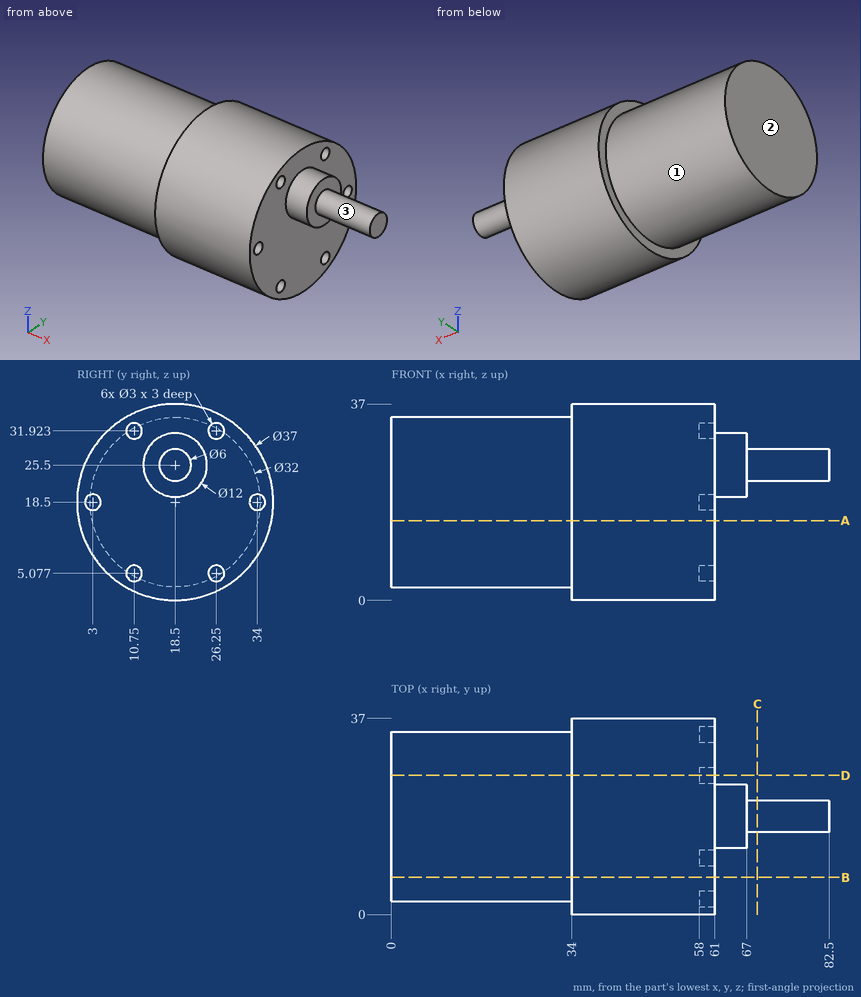
Geometry check sheet. Reference: drawing and pictorial views, mm from the part's lowest x, y, z. A direction names the side the tool comes from. Coordinates: 2 decimals unless noted, no trailing zeros. Loops run counter-clockwise (first coordinate to the right, second up) from the corner with the lowest first, then second, coordinate; pieces in that order, holes last.
1) Sectioned sample at D-D (y = 26.25). Record the boundary of the cut face in (x, z), and give its area (3 significant figures).
2) Sectioned sample at B-B (y = 7). Record the boundary of the cut face in (x, z) (1 decimal), and give its area (3 significant figures).
3) Sectioned sample at C-C (x = 69). Record the boundary of the cut face in (y, z), and give its area (3 significant figures).
4) Gauge pin test, flat ends, axial feed: pin 1 (18.5 mm diameter, centred on y = 22, z = 11, fed in from -X); pin 2 (5 mm diameter, centred on y = 3, z = 18.5, fed in from +X); pin 3 (6 mm diameter, centred on x = 30.5, z = 32, fed in from -Y); pin 4 (10 mm diameter, centred on y = 9, z = 30.5, fed in from +X). Record the tip position at first contact, or that the pin passes through.
5) Access from +Z, -Z, +X, -X, +Y, -Y to the whole of each face (thin tool, end or side, straight path). Record for the marked faces 1, 2 and 3.
6) Sectioned sample at A-A (z = 15). Record the boundary of the cut face in (x, y).
7) Material ranges on probe 1 along X at (y, z) = (20, 18.5); probe 2 along X at (y, z) = (16, 22.5); probe 3 along Y at (x, z) = (57, 35) (1 decimal), recorded low to high.
Check sheet entries:
1. outline: (0, 4.5) - (34, 4.5) - (34, 1.7) - (61, 1.7) - (61, 3.58) - (58, 3.58) - (58, 6.58) - (61, 6.58) - (61, 30.42) - (58, 30.42) - (58, 33.42) - (61, 33.42) - (61, 35.3) - (34, 35.3) - (34, 32.5) - (0, 32.5) - close
1. area: 1,840 mm2
2. outline: (0, 7.4) - (34, 7.4) - (34, 4) - (61, 4) - (61, 33) - (34, 33) - (34, 29.6) - (0, 29.6) - close
2. area: 1,540 mm2
3. outline: circle Ø6 at (18.5, 25.5)
3. area: 28.3 mm2
4. pin 1: stops at x = 0
4. pin 2: stops at x = 61
4. pin 3: stops at y = 6.43
4. pin 4: stops at x = 67
5. face 1: -X
5. face 2: +Z, -Z, -X, +Y, -Y
5. face 3: +X
6. outline: (0, 2.89) - (34, 2.89) - (34, 0.33) - (61, 0.33) - (61, 36.67) - (34, 36.67) - (34, 34.11) - (0, 34.11) - close
7. probe 1: x = 0 to 61
7. probe 2: x = 0 to 67
7. probe 3: y = 10.1 to 26.9
